from build123d import *

# Parameters (mm, degrees)
BOX002_W     = 12
BOX002_H     = 48
BOX002_DEPTH = 4
BOX001_W     = 10
BOX001_H     = 48
BOX001_DEPTH = 12
BOX_W        = 12
BOX_H        = 50
BOX_DEPTH    = 13
FILLET_R     = 3


with BuildPart() as kostka002:
    # Box002 → Box002 (new body)
    with BuildSketch(Plane(origin=(0, 1, 9), x_dir=(1, 0, 0), z_dir=(0, 0, 1))):
        with Locations((6, 24)):
            Rectangle(BOX002_W, BOX002_H)
    extrude(amount=BOX002_DEPTH)


with BuildPart() as kostka001:
    # Box001 → Box001 (new body)
    with BuildSketch(Plane(origin=(1, 1, 1), x_dir=(1, 0, 0), z_dir=(0, 0, 1))):
        with Locations((5, 24)):
            Rectangle(BOX001_W, BOX001_H)
    extrude(amount=BOX001_DEPTH)


with BuildPart() as fillet_body:
    # Box → Box (new body)
    with BuildSketch(Plane.XY):
        with Locations((6, 25)):
            Rectangle(BOX_W, BOX_H)
    extrude(amount=BOX_DEPTH)

    # Cut: cut Kostka001
    add(kostka001.part, mode=Mode.SUBTRACT)

    # Cut001: cut Kostka002
    add(kostka002.part, mode=Mode.SUBTRACT)

    # Fillet
    fillet_edges = [fillet_body.edges().sort_by_distance(p)[0] for p in [
        (0, 0.5, 13),
        (0, 49.5, 13),
        (12, 0.5, 13),
        (12, 49.5, 13),
    ]]
    fillet(fillet_edges, radius=FILLET_R)


solid = fillet_body.part
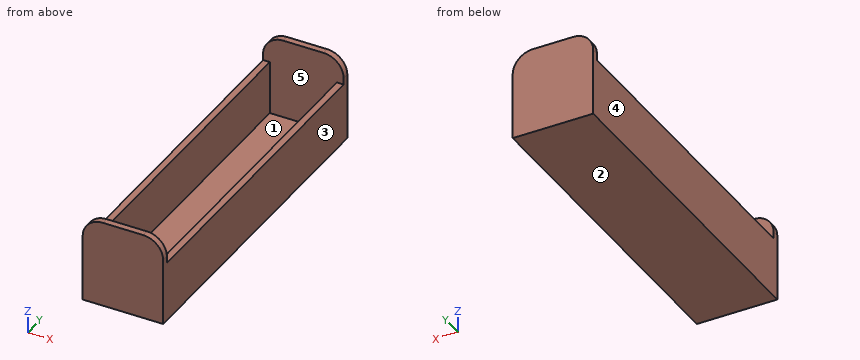
Geometry check sheet. Reference: the model listing, model coordinates, mm. Face numbers are marked on the shaded views. A direction names the side the tool comes from. Give positions to 0.01 mm unless a question says otherwise; leave off trailing zeros. Loops run counter-clockwise (first coordinate to the right, second up) from the corner with the lowest first, then second, coordinate; pieces in that order, holes last. Notation, with made-up numbers: M 36.25,39 L 69.25,39 A23 ccw 69.25,61 Z; hole C 8,87.5 d5. An arc over 180 degrees is marked long. Answer as a JSON object with one key per item and string values. Group by question number.
Item 1: Gauge pin test, flat ends, axial feed: pin 1 (0.5 mm diameter, centred on x = 11.5, y = 24, fed in from +Z); pin 2 (4 mm diameter, centred on x = 8.5, z = 1.5, fed in from -Y); pin 3 (5 mm diameter, centred on x = 6.5, y = 36.5, fed in from +Z). Record the tip position at first contact, or that the pin passes through.
Item 2: Material ranges on L1, parallel to Y at x = 1, z = 9.75; L2, parallel to X at y = 41, z = 5.75; L3, parallel to Z at x = 2, y = 37, recorded low to high.
Item 3: Sectioned sample at B-B on y = 40. Record the boundary of the cut face in (x, z).
Item 4: Mould release check, pull along X, two halves, no side actions. Record for the marked faces 1, 2 and 3: pulls with the +X half, pulls with the -X half, needs draft (parallel to the pull), parting line crosses it, or undercut.
Item 5: Sectioned sample at A-A on z = 2.25. Record the boundary of the cut face in (x, y).
Item 6: Sectioned sample at D-D on z = 11.25. Record the boundary of the cut face in (x, y), plus the area to 3 significant figures.
Item 7: Sectioned sample at C-C on x = 4. Record the boundary of the cut face in (y, z).
Item 8: Access from +Z, -Z, +X, -X, +Y, -Y to the whole of each face (thin tool, end or side, straight path). Record for the marked faces 4 and 5.
Findings below:
{
 "1": {"pin 1": "z = 9", "pin 2": "y = 0", "pin 3": "z = 1"},
 "2": {"L1": "0 to 1, 49 to 50", "L2": "0 to 1, 11 to 12", "L3": "0 to 1"},
 "3": {"outline": "M 0,0 L 12,0 L 12,9 L 11,9 L 11,1 L 1,1 L 1,9 L 0,9 Z"},
 "4": {"face 1": "undercut", "face 2": "needs draft", "face 3": "pulls with the +X half"},
 "5": {"outline": "M 0,0 L 12,0 L 12,50 L 0,50 Z; hole M 1,1 L 11,1 L 11,49 L 1,49 Z"},
 "6": {"outline": "M 0.27,0 L 11.73,0 L 11.73,1 L 0.27,1 Z; M 0.27,49 L 11.73,49 L 11.73,50 L 0.27,50 Z", "area": "22.9 mm2"},
 "7": {"outline": "M 0,0 L 50,0 L 50,13 L 49,13 L 49,1 L 1,1 L 1,13 L 0,13 Z"},
 "8": {"face 4": "+Z, -Z, -X, +Y, -Y", "face 5": "+Z"}
}
